Can you work these out from the drawing? Everything is in mm from the part's minimum corner. A direction names the side the tool comes from. Round coordinates to 2 decimals unless told otherwise and drop trailing zeros. Loops run counter-clockwise (first coordinate to the right, second up) from the corner with the lowest first, then second, coordinate; pieces in that order, holes last. Notation, with made-up numbers: (-30, 26.25) - (14, 26.25) arc R14 cw to (14, 40.25) - close; hole circle Ø3 at (27.25, 29.25). An arc over 180 degrees is marked (long way). Answer as CSV lines item,"result". Start each with the question number.
1) Suppose I cut it at C-C, the plane y = 10.5. Write out the boundary of the cut face in (x, z).
2) We'd pull the mould along Z, two halves only. Please class the marked faces 6, 7, 8 and 9: pulls with the +Z half, pulls with the -Z half, needs draft (parallel to the pull), parting line crosses it, or undercut.
3) Suppose I cut it at B-B, the plane z = 70. Write out the boundary of the cut face in (x, y).
4) Suppose I cut it at D-D, the plane y = 44. Write out the boundary of the cut face in (x, z).
5) Which directions (+Z, -Z, +X, -X, +Y, -Y) give clear straight access to the entire face, cutting with the end or side of a thin tool? Please do the marked faces 1, 2, 3, 4 and 5.
6) Please list where these lines run through material, in increasing order: line 1 along X through (y, z) = (85.05, 66); line 2 along X through (y, z) = (39.5, 36); line 3 along Z through (x, y) = (73, 84.25).
7) I'm going to push flat-ended pins straight in: pin 1 Ø13 at (x, z) = (33, 54) entering from -Y; pin 2 Ø3 at (y, z) = (62.5, 8) entering from -X (1 decimal); pin 3 Ø6 at (x, y) = (10.5, 24.5) entering from +Z; pin 4 Ø3 at (x, z) = (22.5, 9) entering from +Y. Where does each tip first touch, or does it pass through?
8) Suppose I cut it at A-A, the plane x = 29.5. Write out the boundary of the cut face in (y, z) (1 decimal).
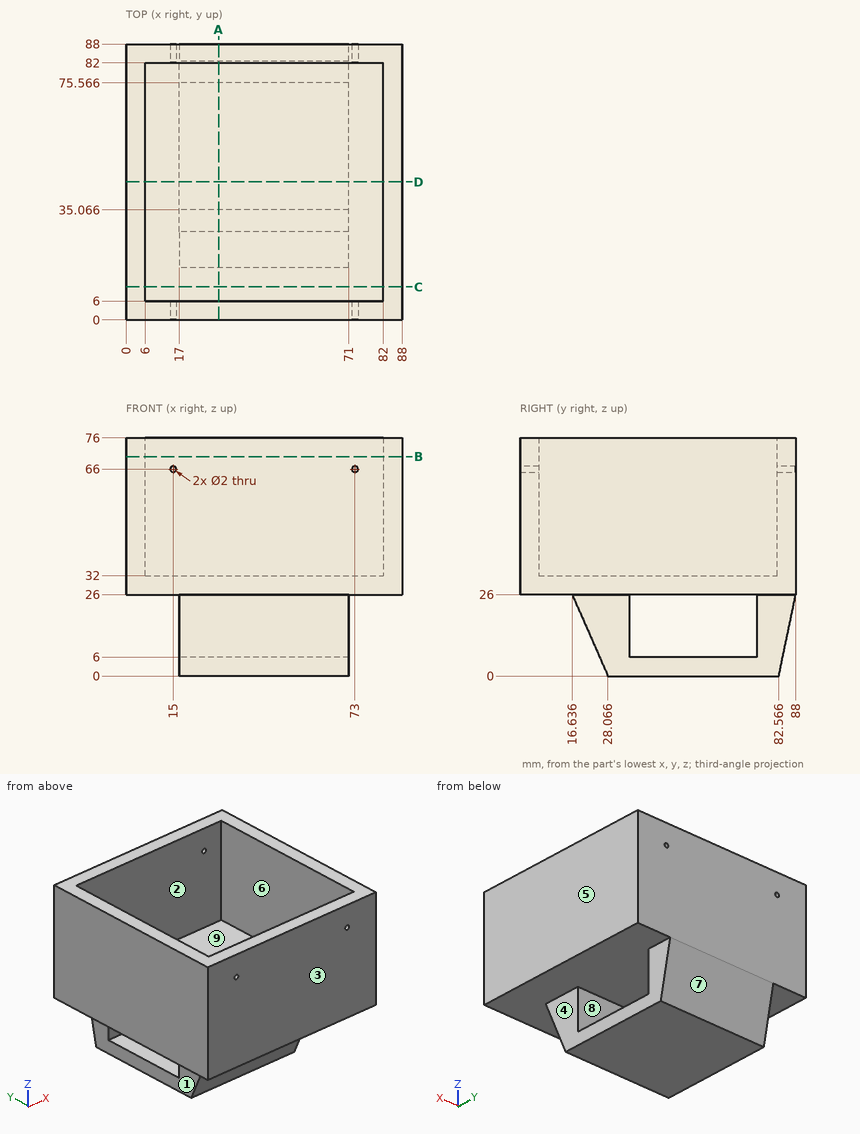
Filled sheet:
1,outline,"(0, 26) - (88, 26) - (88, 76) - (82, 76) - (82, 32) - (6, 32) - (6, 76) - (0, 76) - close"
2,face 6,"needs draft"
2,face 7,"pulls with the -Z half"
2,face 8,"undercut"
2,face 9,"pulls with the +Z half"
3,outline,"(0, 0) - (88, 0) - (88, 88) - (0, 88) - close; hole (6, 6) - (82, 6) - (82, 82) - (6, 82) - close"
4,outline,"(0, 26) - (88, 26) - (88, 76) - (82, 76) - (82, 32) - (6, 32) - (6, 76) - (0, 76) - close; (17, 0) - (71, 0) - (71, 6) - (17, 6) - close"
5,face 1,"-Z, -X, +Y, -Y"
5,face 2,"+Z"
5,face 3,"+Z, -Z, +X, -X, -Y"
5,face 4,"-Z, +X, +Y, -Y"
5,face 5,"+Z, -Z, +X, +Y, -Y"
6,line 1,"0 to 14, 16 to 72, 74 to 88"
6,line 2,"0 to 6, 82 to 88"
6,line 3,"26 to 65, 67 to 76"
7,pin 1,"y = 0"
7,pin 2,"through"
7,pin 3,"z = 32"
7,pin 4,"y = 84.76"
8,outline,"(0, 26) - (16.6, 26) - (28.1, 0) - (82.6, 0) - (88, 26) - (88, 76) - (82, 76) - (82, 32) - (6, 32) - (6, 76) - (0, 76) - close; hole (35.1, 6) - (75.6, 6) - (75.6, 26) - (35.1, 26) - close"
